```python
from build123d import *

# Parameters (mm, degrees)
F3_R     = 2
F4_DEPTH = 1.6


with BuildPart() as f1:
    # F0 (on Front) → F1 (revolve)
    with BuildSketch(Plane.XZ):
        Polygon((2, 0), (0, 0), (0, -16.5), (3.8, -16.5), (3.8, -1.8), (4.7, -1.8), (4.7, 0), (3, 0), (3, 3), (2, 3), align=None)
    revolve(axis=Axis((0, 0, -8.25), (0, 0, 1)))

    # F3 (on offset) → F4 (join)
    with BuildSketch(Plane.XY.offset(1)):
        Polygon((4.5, -2.598076), (4.5, 2.598076), (0, 5.196152), (-4.5, 2.598076), (-4.5, -2.598076), (0, -5.196152), align=None)
        Circle(F3_R, mode=Mode.SUBTRACT)
    extrude(amount=F4_DEPTH)


solid = f1.part
```
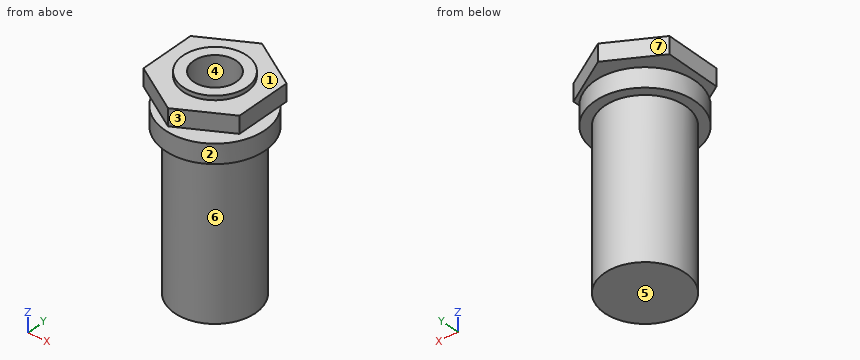
Build history of the part. All positions in model axes, mm. Face numbers are marked on the shaded views. A direction names the side the tool comes from. Give positions to 0.01 mm unless a question says otherwise; leave off trailing zeros. Loops run counter-clockwise (first coordinate to the right, second up) from the corner with the lowest first, then second, coordinate; pieces in that order, holes last. Notation, with made-up numbers: (49.5, 74) -> (63.5, 74) arc R29 cw to (63.5, 109) -> close; hole circle Ø7 at (33.25, 80). An arc over 180 degrees is marked (long way). One line per question, with ' | ' between items. Start each with the question number.
1) Cut at D-D (z = -5.25). Give the cut face in (x, y).
2) Cut at B-B (y = 0). Give the cut face in (x, z).
3) Probe L1, parallel to Z at x = 4, y = 1.25; L2, parallel to Z at x = 2.75, y = 2.25; L3, parallel to Y at x = 0, z = 0.75. List the from-to ranges inside material, lowest first.
4) Two-plate mould, pull along X, no slides. Class the marked faces 1, 2, 3 and 4: released by +X, released by -X, zero draft, split by the parting line, or undercut.
5) Pin check, flat tips, straight feed: pin 1 (0.8 mm diameter, centred on y = 0, z = 2, fed in from +X); pin 2 (0.5 mm diameter, centred on y = 0, z = 1.5, fed in from -X); pin 3 (3 mm diameter, centred on x = 0, y = 0, fed in from +Z). Stop position of each tip, or through.
6) Cut at A-A (x = -3.25). Give the cut face in (y, z).
7) Cut at C-C (x = 1). Give the cut face in (y, z).
8) 3-axis set-ups, long thin cutter, end or side, ignore diameter. For the marked faces 5, 6 and 7: which of +Z, -Z, +X, -X, +Y, -Y reach the whole face in a straight line?
Return value:
1) outline: circle Ø7.6 at (0, 0)
2) outline: (-4.7, -1.8) -> (-3.8, -1.8) -> (-3.8, -16.5) -> (3.8, -16.5) -> (3.8, -1.8) -> (4.7, -1.8) -> (4.7, 0) -> (3, 0) -> (3, 1) -> (4.5, 1) -> (4.5, 2.6) -> (3, 2.6) -> (3, 3) -> (2, 3) -> (2, 0) -> (-2, 0) -> (-2, 3) -> (-3, 3) -> (-3, 2.6) -> (-4.5, 2.6) -> (-4.5, 1) -> (-3, 1) -> (-3, 0) -> (-4.7, 0) -> close
3) L1: -1.8 to 0, 1 to 2.6 | L2: -16.5 to 0, 1 to 2.6 | L3: -3 to -2, 2 to 3
4) face 1: zero draft | face 2: split by the parting line | face 3: released by +X | face 4: undercut
5) pin 1: x = 4.5 | pin 2: x = -4.5 | pin 3: z = 0
6) outline: (-3.4, -1.8) -> (-1.97, -1.8) -> (-1.97, -16.5) -> (1.97, -16.5) -> (1.97, -1.8) -> (3.4, -1.8) -> (3.4, 0) -> (-3.4, 0) -> close; (-3.32, 1) -> (3.32, 1) -> (3.32, 2.6) -> (-3.32, 2.6) -> close
7) outline: (-4.62, 1) -> (-2.83, 1) -> (-2.83, 0) -> (-4.59, 0) -> (-4.59, -1.8) -> (-3.67, -1.8) -> (-3.67, -16.5) -> (3.67, -16.5) -> (3.67, -1.8) -> (4.59, -1.8) -> (4.59, 0) -> (2.83, 0) -> (2.83, 1) -> (4.62, 1) -> (4.62, 2.6) -> (2.83, 2.6) -> (2.83, 3) -> (1.73, 3) -> (1.73, 0) -> (-1.73, 0) -> (-1.73, 3) -> (-2.83, 3) -> (-2.83, 2.6) -> (-4.62, 2.6) -> close
8) face 5: -Z, +X, -X, +Y, -Y | face 6: -Z | face 7: +Z, -X, +Y
